from build123d import *

# Parameters (mm, degrees)
SKETCH2_R           = 1.112004448
BOSS_EXTRUDE1_DEPTH = 0.5
SKETCH3_W           = 0.5
SKETCH3_H           = 41.135021261
BOSS_EXTRUDE2_DEPTH = 0.15
SKETCH4_W           = 1.5
SKETCH4_H           = 1.027696227
BOSS_EXTRUDE3_DEPTH = 1


with BuildPart() as part:
    # Sketch2 → Boss-Extrude1 (new body)
    with BuildSketch(Plane.XY):
        Polygon((-10, 13.571131009), (10, 13.571131009), (10, 54.708363732), (8.281546087, 56.925194639), (8.281546087, 64.240363418), (10, 66.862498938), (10, 72.571131009), (-10, 72.571131009), (-10, 66.862498938), (-8.281546087, 64.240363418), (-8.281546087, 56.925194639), (-10, 54.708363732), align=None)
        with Locations((8.618613348, 71.214744162)):
            Circle(SKETCH2_R, mode=Mode.SUBTRACT)
        with Locations((-8.618613348, 71.214744162)):
            Circle(SKETCH2_R, mode=Mode.SUBTRACT)
    extrude(amount=BOSS_EXTRUDE1_DEPTH)

    # Sketch3 → Boss-Extrude2 (add)
    with BuildSketch(Plane.XY.offset(0.5)):
        with Locations((-9.5, 34.13864164)):
            Rectangle(SKETCH3_W, SKETCH3_H)
        with Locations((-8.5, 34.13864164)):
            Rectangle(SKETCH3_W, SKETCH3_H)
        with Locations((-7.5, 34.13864164)):
            Rectangle(SKETCH3_W, SKETCH3_H)
        with Locations((-6.5, 34.13864164)):
            Rectangle(SKETCH3_W, SKETCH3_H)
        with Locations((-5.5, 34.13864164)):
            Rectangle(SKETCH3_W, SKETCH3_H)
        with Locations((-4.5, 34.13864164)):
            Rectangle(SKETCH3_W, SKETCH3_H)
        with Locations((-3.5, 34.13864164)):
            Rectangle(SKETCH3_W, SKETCH3_H)
        with Locations((-2.5, 34.13864164)):
            Rectangle(SKETCH3_W, SKETCH3_H)
        with Locations((-1.5, 34.13864164)):
            Rectangle(SKETCH3_W, SKETCH3_H)
        with Locations((-0.5, 34.13864164)):
            Rectangle(SKETCH3_W, SKETCH3_H)
        with Locations((0.5, 34.13864164)):
            Rectangle(SKETCH3_W, SKETCH3_H)
        with Locations((1.5, 34.13864164)):
            Rectangle(SKETCH3_W, SKETCH3_H)
        with Locations((2.5, 34.13864164)):
            Rectangle(SKETCH3_W, SKETCH3_H)
        with Locations((3.5, 34.13864164)):
            Rectangle(SKETCH3_W, SKETCH3_H)
        with Locations((4.5, 34.13864164)):
            Rectangle(SKETCH3_W, SKETCH3_H)
        with Locations((5.5, 34.13864164)):
            Rectangle(SKETCH3_W, SKETCH3_H)
        with Locations((6.5, 34.13864164)):
            Rectangle(SKETCH3_W, SKETCH3_H)
        with Locations((7.5, 34.13864164)):
            Rectangle(SKETCH3_W, SKETCH3_H)
        with Locations((8.5, 34.13864164)):
            Rectangle(SKETCH3_W, SKETCH3_H)
        with Locations((9.5, 34.13864164)):
            Rectangle(SKETCH3_W, SKETCH3_H)
    extrude(amount=BOSS_EXTRUDE2_DEPTH)

    # Sketch4 → Boss-Extrude3 (add)
    with BuildSketch(Plane.XY.offset(0.5)):
        with Locations((-0.75, 71.676816486)):
            Rectangle(SKETCH4_W, SKETCH4_H)
        with Locations((0.75, 71.676816486)):
            Rectangle(SKETCH4_W, SKETCH4_H)
    extrude(amount=BOSS_EXTRUDE3_DEPTH)


solid = part.part
Input: part model. Units: mm. Frame: model coordinates. A direction names the side the tool comes from. Coordinates: 2 decimals unless noted, no trailing zeros. Order: outer loops, then holes, each group sorted by start corner. A loop starts at its lowest first (then second) coordinate and runs counter-clockwise, first axis right, second up. Notation, with made-up numbers: M 35.25,39.5 L 79.25,39.5 A24 cw 79.25,66.5 Z; hole C -18,67.25 d6. An arc over 180 degrees is marked long. Write item = value, one per line. Start each with the question number.
(1) First-contact query: P1, Ø0.6, axis at y = 59.5, z = 0, coming from the +X side; P2, Ø10, axis at x = 4, y = 37, coming from the +Z side. Flat tips, straight axial feed; report the tip coordinate or a pass-through.
(2) Section B-B on z = 1.1. Output: boundary loops of the cut face in (x, y).
(3) Pull-direction query (X, two-part tool) for faces 5 (the flat face through (0, 50, 0.5)), 6 (the cylindrical face through (-8.763, 72.317, 0.246)), 7 (the flat face through (9.153, 55.801, 0.246)), 8 (the flat face through (-9.153, 65.57, 0.246)); classes: released by +X, released by -X, zero draft, split by the parting line, or undercut.
(4) Section A-A on y = 69.5. Output: boundary loops of the cut face in (x, z), and give its area (3 significant figures).
(5) Line query: line 1 along Y through (x, z) = (0.75, 0.65); line 2 along Z through (x, y) = (-4.75, 70); line 3 along Y through (x, z) = (-8.75, 0.4). Output: solid intervals per line, ascending. Write a range as [from, to].
(6) Reachability of faces 1 (the flat face through (-9.13, 55.83, 0.25)), 2 (the flat face through (0, 72.191, 1)), 3 (the flat face through (0, 72, 1.5)), 4 (the flat face through (9.129, 65.533, 0.246)) from +Z, -Z, +X, -X, +Y, -Y: full face, straight path, thin tool, end or side. Return the list, or none.
Result set:
q1.P1 = 8.28
q1.P2 = 0.65
q2.outline = M -1.5,71.16 L 1.5,71.16 L 1.5,72.19 L -1.5,72.19 Z
q3.face_5 = undercut
q3.face_6 = undercut
q3.face_7 = released by +X
q3.face_8 = released by -X
q4.outline = M -10,0 L 10,0 L 10,0.5 L -10,0.5 Z
q4.area = 10.0 mm²
q5.line_1 = [71.16, 72.19]
q5.line_2 = [0, 0.5]
q5.line_3 = [13.57, 56.32], [64.96, 70.11], [72.32, 72.57]
q6.face_1 = +Z, -Z, -X
q6.face_2 = +Z, +X, -X, +Y
q6.face_3 = +Z, +X, -X, +Y, -Y
q6.face_4 = +Z, -Z, +X
